```python
from build123d import *

# Parameters (mm, degrees)
SKETCH_1_W          = 80
SKETCH_1_H          = 62
EXTRUDE_1_DEPTH     = 4
FILLET_1_R          = 4
FILLET_2_R          = 4
SKETCH_2_R          = 1.6
CUT_EXTRUDE_1_DEPTH = 10
SKETCH_3_R          = 1.6
CUT_EXTRUDE_2_DEPTH = 10
CUT_EXTRUDE_3_DEPTH = 10
FILLET_3_R          = 3
CUT_EXTRUDE_4_DEPTH = 10
FILLET_4_R          = 3


with BuildPart() as part:
    # 草图1 → 凸台-拉伸1 (new body)
    with BuildSketch(Plane.XY):
        Rectangle(SKETCH_1_W, SKETCH_1_H)
    extrude(amount=EXTRUDE_1_DEPTH)

    # 圆角1
    fillet_1_edges = [part.edges().sort_by_distance(p)[0] for p in [
        (-40, -31, 2),
        (-40, 31, 2),
    ]]
    fillet(fillet_1_edges, radius=FILLET_1_R)

    # 圆角2
    fillet_2_edges = [part.edges().sort_by_distance(p)[0] for p in [
        (40, -31, 2),
        (40, 31, 2),
    ]]
    fillet(fillet_2_edges, radius=FILLET_2_R)

    # 草图2 → 切除-拉伸1 (cut)
    with BuildSketch(Plane.XY.offset(4)):
        with Locations((11, -19)):
            Circle(SKETCH_2_R)
        with Locations((31, -19)):
            Circle(SKETCH_2_R)
        with Locations((35, 6.5)):
            Circle(SKETCH_2_R)
        with Locations((15, 6.5)):
            Circle(SKETCH_2_R)
        with Locations((11, 19)):
            Circle(SKETCH_2_R)
        with Locations((31, 19)):
            Circle(SKETCH_2_R)
        with Locations(Location((15, -6.5, 0), (0, 0, 180))):
            Circle(SKETCH_2_R)
        with Locations(Location((35, -6.5, 0), (0, 0, 180))):
            Circle(SKETCH_2_R)
    extrude(amount=-CUT_EXTRUDE_1_DEPTH, mode=Mode.SUBTRACT)

    # 草图3 → 切除-拉伸2 (cut)
    with BuildSketch(Plane.XY.offset(4)):
        with Locations((-36, -27)):
            Circle(SKETCH_3_R)
        with Locations((-36, 27)):
            Circle(SKETCH_3_R)
    extrude(amount=-CUT_EXTRUDE_2_DEPTH, mode=Mode.SUBTRACT)

    # 草图4 → 切除-拉伸3 (cut)
    with BuildSketch(Plane.XY.offset(4)):
        Polygon((-12.535533906, 0), (-34, 21.464466094), (-34, -21.464466094), align=None)
        Polygon((5.93014286, 25), (-30.464466094, 25), (-7.964466094, 2.5), (13.13014286, 2.5), align=None)
        Polygon((-7.964466094, -2.5), (-30.464466094, -25), (5.93014286, -25), (13.13014286, -2.5), align=None)
    extrude(amount=-CUT_EXTRUDE_3_DEPTH, mode=Mode.SUBTRACT)

    # 圆角3
    fillet_3_edges = [part.edges().sort_by_distance(p)[0] for p in [
        (-7.964466094, -2.5, 2),
        (13.13014286, -2.5, 2),
        (5.93014286, -25, 2),
        (-30.464466094, -25, 2),
        (-30.464466094, 25, 2),
        (5.93014286, 25, 2),
        (13.13014286, 2.5, 2),
        (-7.964466094, 2.5, 2),
        (-12.535533906, 0, 2),
        (-34, -21.464466094, 2),
        (-34, 21.464466094, 2),
    ]]
    fillet(fillet_3_edges, radius=FILLET_3_R)

    # 草图5 → 切除-拉伸4 (cut)
    with BuildSketch(Plane.XY.offset(4)):
        Polygon((33.13014286, -2.5), (19.42985714, -2.5), (12.22985714, -25), (25.93014286, -25), align=None)
        Polygon((25.93014286, 25), (12.22985714, 25), (19.42985714, 2.5), (33.13014286, 2.5), align=None)
    extrude(amount=-CUT_EXTRUDE_4_DEPTH, mode=Mode.SUBTRACT)

    # 圆角4
    fillet_4_edges = [part.edges().sort_by_distance(p)[0] for p in [
        (19.42985714, -2.5, 2),
        (33.13014286, -2.5, 2),
        (25.93014286, -25, 2),
        (12.22985714, -25, 2),
        (19.42985714, 2.5, 2),
        (12.22985714, 25, 2),
        (25.93014286, 25, 2),
        (33.13014286, 2.5, 2),
    ]]
    fillet(fillet_4_edges, radius=FILLET_4_R)


solid = part.part
```
Read the model definition and answer for the solid it produces. Units are mm, in the model's axes. A direction names the side the tool comes from. Round coordinates to 2 decimals unless told otherwise and drop trailing zeros. Write each loop counter-clockwise with the first axis right and the second up, starting at its lowest first coordinate (ties: lowest second). Pieces come first, ordered by that corner, then holes. Notation, with made-up numbers: (-2.5, 2.5) -> (17.5, 2.5) arc R17 cw to (17.5, 30.5) -> close; hole circle Ø5 at (-25, 8). An arc over 180 degrees is marked (long way). Answer in a Markdown table with one row per item. Add a question column.
1) Determine the mould class of faces 1 (the face through (-38.859, 29.797, 2.028)), 2 (the face through (25, 2.5, 2)), 3 (the face through (40, 0, 2)), 4 (the face through (38.797, -29.859, 2.028)) for opening direction Y: pulls with the +Y half, pulls with the -Y half, needs draft (parallel to the pull), parting line crosses it, or undercut.
2) Find section D-D, the plane y = 15.5. Determine the outline of the cut face in (x, z).
3) Find section C-C, the plane x = 14.5. Determine the outline of the cut face in (y, z).
4) Which of the six approach directions +Z, -Z, +X, -X, +Y, -Y give full straight-line access (tool end or side, diameter ignored) to faces 5 (the face through (-40, 0, 2)), 6 (the face through (20, -25, 2))?
5) Consider line 1 (Y direction, x = 2, z = 3.4); line 2 (Y direction, x = -10, z = 2.95); line 3 (X direction, y = -11, z = 1). Determine where each line is inside the solid, lowest interval first.
6) Find section A-A, the plane y = 0. Determine the outline of the cut face in (x, z).
7) Find section B-B, the plane x = 22.5. Determine the outline of the cut face in (y, z), and give its area (3 significant figures).
Findings below:
| question | item | result |
|---|---|---|
| 1 | face 1 | pulls with the +Y half |
| 1 | face 2 | undercut |
| 1 | face 3 | needs draft |
| 1 | face 4 | pulls with the -Y half |
| 2 | outline | (-40, 0) -> (-33.71, 0) -> (-33.71, 4) -> (-40, 4) -> close; (-28.04, 0) -> (-20.96, 0) -> (-20.96, 4) -> (-28.04, 4) -> close; (8.97, 0) -> (15.27, 0) -> (15.27, 4) -> (8.97, 4) -> close; (28.97, 0) -> (40, 0) -> (40, 4) -> (28.97, 4) -> close |
| 3 | outline | (-31, 0) -> (-24.37, 0) -> (-24.37, 4) -> (-31, 4) -> close; (-17.91, 0) -> (-8.02, 0) -> (-8.02, 4) -> (-17.91, 4) -> close; (-4.98, 0) -> (4.98, 0) -> (4.98, 4) -> (-4.98, 4) -> close; (8.02, 0) -> (17.91, 0) -> (17.91, 4) -> (8.02, 4) -> close; (24.37, 0) -> (31, 0) -> (31, 4) -> (24.37, 4) -> close |
| 4 | face 5 | +Z, -Z, -X, +Y, -Y |
| 4 | face 6 | +Z, -Z |
| 5 | line 1 | -31 to -25, -2.5 to 2.5, 25 to 31 |
| 5 | line 2 | -31 to -25, -4.54 to 4.54, 25 to 31 |
| 5 | line 3 | -40 to -34, -23.54 to -16.46, 10.41 to 16.71, 30.41 to 40 |
| 6 | outline | (-40, 0) -> (-34, 0) -> (-34, 4) -> (-40, 4) -> close; (-13.78, 0) -> (40, 0) -> (40, 4) -> (-13.78, 4) -> close |
| 7 | outline | (-31, 0) -> (-25, 0) -> (-25, 4) -> (-31, 4) -> close; (-2.5, 0) -> (2.5, 0) -> (2.5, 4) -> (-2.5, 4) -> close; (25, 0) -> (31, 0) -> (31, 4) -> (25, 4) -> close |
| 7 | area | 68.0 mm² |
